```python
from build123d import *

# Parameters (mm, degrees)
SKETCH1_W           = 300
SKETCH1_H           = 240
SKETCH1_R           = 2
BOSS_EXTRUDE1_DEPTH = 3


with BuildPart() as part:
    # Sketch1 → Boss-Extrude1 (new body)
    with BuildSketch(Plane.XY):
        Rectangle(SKETCH1_W, SKETCH1_H)
        with Locations((-95, 110)):
            Circle(SKETCH1_R, mode=Mode.SUBTRACT)
        with Locations((95, 110)):
            Circle(SKETCH1_R, mode=Mode.SUBTRACT)
        with Locations(Location((95, -110, 0), (0, 0, 180))):
            Circle(SKETCH1_R, mode=Mode.SUBTRACT)
        with Locations(Location((-95, -110, 0), (0, 0, 180))):
            Circle(SKETCH1_R, mode=Mode.SUBTRACT)
        Polygon((99, 101), (99, -101), (91, -94.6), (91, 94.6), align=None, mode=Mode.SUBTRACT)
        Polygon((82, 112.5), (-82, 112.5), (-75.75, 107.5), (75.75, 107.5), align=None, mode=Mode.SUBTRACT)
    extrude(amount=BOSS_EXTRUDE1_DEPTH)


solid = part.part
```
Here's how the part is built. I have some questions about the finished solid (model axes, mm). Give positions to 0.01 mm unless a question says otherwise; leave off trailing zeros. Order: outer loops, then holes, each group sorted by start corner. A loop starts at its lowest first (then second) coordinate and runs counter-clockwise, first axis right, second up. Notation, with made-up numbers: M -9.5,27.5 L 38.5,27.5 A20 ccw 38.5,33.5 Z; hole C 2.25,-13.5 d7. An arc over 180 degrees is marked long. Use a Markdown table: item, result. Add a question column.
1. Suppose I cut it at B-B (x = 46.5). List the corners of the cut face in (y, z) for me, and give its area (3 significant figures).
2. Suppose I cut it at C-C (z = 1.3). List the corners of the cut face in (x, y) for me, and give its area (3 significant figures).
3. Suppose I cut it at A-A (y = -54). List the corners of the cut face in (x, z) for me, and give its area (3 significant figures).
4. I need wall thicknesses on probe 1 along Y at (x, z) = (-95, 1.9); probe 2 along X at (y, z) = (-110, 2.3); probe 3 along X at (y, z) = (-77, 2). Which ranges of each line are inside material? Lowest first, please. Write a range as from..to.
5. If we mould it in two halves opening along Y, with no side actions, what happens to faces 1 (the flat face through (95.056, -97.845, 1.479)), 2 (the flat face through (-2, 2, 3))? For each: +Y half, -Y half, draft (parallel to the pull), parting line (faces both ways), or undercut.
Results list:
| question | item | result |
|---|---|---|
| 1 | outline | M -120,0 L 107.5,0 L 107.5,3 L -120,3 Z; M 112.5,0 L 120,0 L 120,3 L 112.5,3 Z |
| 1 | area | 705 mm² |
| 2 | outline | M -150,-120 L 150,-120 L 150,120 L -150,120 Z; hole C -95,-110 d4; hole C -95,110 d4; hole M -82,112.5 L -75.75,107.5 L 75.75,107.5 L 82,112.5 Z; hole M 91,-94.6 L 99,-101 L 99,101 L 91,94.6 Z; hole C 95,-110 d4; hole C 95,110 d4 |
| 2 | area | 69,600 mm² |
| 3 | outline | M -150,0 L 91,0 L 91,3 L -150,3 Z; M 99,0 L 150,0 L 150,3 L 99,3 Z |
| 3 | area | 876 mm² |
| 4 | probe 1 | y = -120..-112, -108..108, 112..120 |
| 4 | probe 2 | x = -150..-97, -93..93, 97..150 |
| 4 | probe 3 | x = -150..91, 99..150 |
| 5 | face 1 | undercut |
| 5 | face 2 | draft |
